Could you check a few things on this model? Use its own coordinates, in mm. Face numbers are marked on the shaded views. A direction names the side the tool comes from. Give positions to 0.01 mm unless a question says otherwise; leave off trailing zeros. Write each question's results on one line, items separated by ' | '. Start each with the question number.
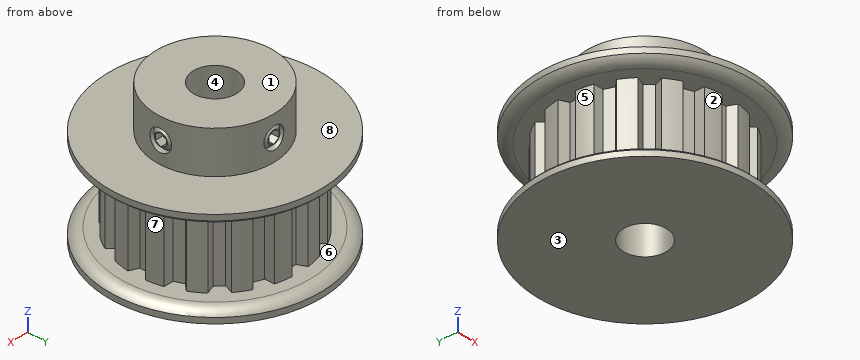
```python
from build123d import *

# Parameters (mm, degrees)
CUT_EXTRUDE1_START = 2.2987
CUT_EXTRUDE1_DEPTH = 10.922
CIRPATTERN1_COUNT  = 16
SKETCH4_R          = 1.5875
CUT_EXTRUDE2_DEPTH = 25.705805871
CUT_EXTRUDE3_DEPTH = 1.190625
CIRPATTERN2_COUNT  = 2
CIRPATTERN2_ANGLE  = 90


with BuildPart() as part:
    # Sketch2 → Revolve1 (revolve)
    with BuildSketch(Plane(origin=(0, 0, 0), x_dir=(0, 0, -1), z_dir=(1, 0, 0)), mode=Mode.PRIVATE) as revolve1_sk:
        with BuildLine():
            Line((-10.3124, 3.175), (10.3124, 3.175))
            Line((10.3124, 3.175), (10.3124, 15.875))
            Line((10.3124, 15.875), (9.46785, 15.875))
            ThreePointArc((9.46785, 15.875), (8.846219323, 15.130824061), (8.6233, 14.187145354))
            Line((8.6233, 14.187145354), (8.6233, 12.499290707))
            Line((8.6233, 12.499290707), (-2.2987, 12.499290707))
            Line((-2.2987, 12.499290707), (-2.2987, 14.187145354))
            ThreePointArc((-2.2987, 14.187145354), (-2.521619323, 15.130824061), (-3.14325, 15.875))
            Line((-3.14325, 15.875), (-3.9878, 15.875))
            Line((-3.9878, 15.875), (-3.9878, 8.7376))
            Line((-3.9878, 8.7376), (-10.3124, 8.7376))
            Line((-10.3124, 8.7376), (-10.3124, 3.175))
        make_face()
    revolve(revolve1_sk.sketch.rotate(Axis((0, 0, 10.3124), (0, 0, -1)), 90), axis=Axis((0, 0, 10.3124), (0, 0, -1)))

    # Sketch3 → Cut-Extrude1 (cut)
    with BuildSketch(Plane.XY.offset(CUT_EXTRUDE1_START)):
        with BuildLine():
            Line((-0.690489274, 11.1633), (0.690489274, 11.1633))
            Line((0.690489274, 11.1633), (1.2827, 12.4333))
            ThreePointArc((1.2827, 12.4333), (0, 12.499290707), (-1.2827, 12.4333))
            Line((-1.2827, 12.4333), (-0.690489274, 11.1633))
        make_face()
    cut_extrude1 = extrude(amount=-CUT_EXTRUDE1_DEPTH, mode=Mode.SUBTRACT)

    # CirPattern1: Cut-Extrude1 ×16 about axis
    cirpattern1_axis = Axis((0, 0, 0), (0, 0, 1))
    for i in range(1, CIRPATTERN1_COUNT):
        add(cut_extrude1.rotate(cirpattern1_axis, i * 360 / CIRPATTERN1_COUNT), mode=Mode.SUBTRACT)

    # Sketch4 → Cut-Extrude2 (cut, through all)
    with BuildSketch(Plane(origin=(0, 0, 0), x_dir=(1, 0, 0), z_dir=(0, 1, 0))):
        with Locations(Location((0, -7.1501, 0), (0, 0, 90))):
            Circle(SKETCH4_R)
    cut_extrude2 = extrude(amount=CUT_EXTRUDE2_DEPTH, mode=Mode.SUBTRACT)

    # Sketch5 → Revolve2 (revolve)
    with BuildSketch(Plane.XY.offset(7.1501), mode=Mode.PRIVATE) as revolve2_sk:
        Polygon((0, 8.592176529), (0, 3.175), (-0.9525, 3.175), (-1.5875, 3.81), (-1.5875, 7.957176529), (-0.9525, 8.592176529), align=None)
    revolve2 = revolve(revolve2_sk.sketch.rotate(Axis((0, 0, 7.1501), (0, 1, 0)), 270), axis=Axis((0, 0, 7.1501), (0, 1, 0)))

    # Sketch6 → Cut-Extrude3 (cut)
    with BuildSketch(Plane(origin=(0, 8.592176529, 0), x_dir=(-1, 0, 0), z_dir=(0, -1, 0))):
        Polygon((0, -6.233556448), (-0.79375, -6.691828224), (-0.79375, -7.608371776), (0, -8.066643552), (0.79375, -7.608371776), (0.79375, -6.691828224), align=None)
    cut_extrude3 = extrude(amount=CUT_EXTRUDE3_DEPTH, mode=Mode.SUBTRACT)

    # CirPattern2: Cut-Extrude2, Revolve2, Cut-Extrude3 ×2 about axis
    cirpattern2_axis = Axis((0, 0, 0), (0, 0, -1))
    add([cut_extrude2.rotate(cirpattern2_axis, i * CIRPATTERN2_ANGLE / (CIRPATTERN2_COUNT - 1)) for i in range(1, CIRPATTERN2_COUNT)], mode=Mode.SUBTRACT)
    add([revolve2.rotate(cirpattern2_axis, i * CIRPATTERN2_ANGLE / (CIRPATTERN2_COUNT - 1)) for i in range(1, CIRPATTERN2_COUNT)])
    add([cut_extrude3.rotate(cirpattern2_axis, i * CIRPATTERN2_ANGLE / (CIRPATTERN2_COUNT - 1)) for i in range(1, CIRPATTERN2_COUNT)], mode=Mode.SUBTRACT)


solid = part.part
```
Q1. Which directions (+Z, -Z, +X, -X, +Y, -Y) give clear straight access to the entire face, cutting with the end or side of a thin tool? Please do the marked faces 4, 5, 6, 7 and 8.
Q2. If we mould it in two halves opening along Z, with no side actions, what happens to the marked faces 1, 2 and 3? For each: +Z half, -Z half, draft (parallel to the pull), parting line (faces both ways), or undercut.
Q3. I'm going to push flat-ended pins straight in: pin 1 Ø2.5 at (x, z) = (0, 7.15) entering from +Y; pin 2 Ø1 at (x, y) = (-6.5, -12) entering from +Z; pin 3 Ø3 at (x, z) = (7.5, -2.5) entering from +Y; pin 4 Ø8 at (y, z) = (1, 4) entering from +X (3 decimals). Where does each tip first touch, or does it pass through?
Q4. I need wall thicknesses on L1, parallel to Z at x = 11, y = -6; L2, parallel to Y at x = -10.5, z = -2; L3, parallel to Z at x = -6.5, y = 9. Which ranges of each line are inside material? Lowest first, please. Write a range as from..to.
Conclusion:
1) face 4: +Z, -Z | face 5: -X, -Y | face 6: none | face 7: +X, +Y | face 8: +Z
2) face 1: +Z half | face 2: undercut | face 3: -Z half
3) pin 1: y = 8.59 | pin 2: z = 3.99 | pin 3: y = 10.97 | pin 4: x = 15.875
4) L1: -10.31..-8.62, 2.3..3.99 | L2: -6.78..-5.4, -3.82..3.82, 5.4..6.78 | L3: -10.31..3.99
